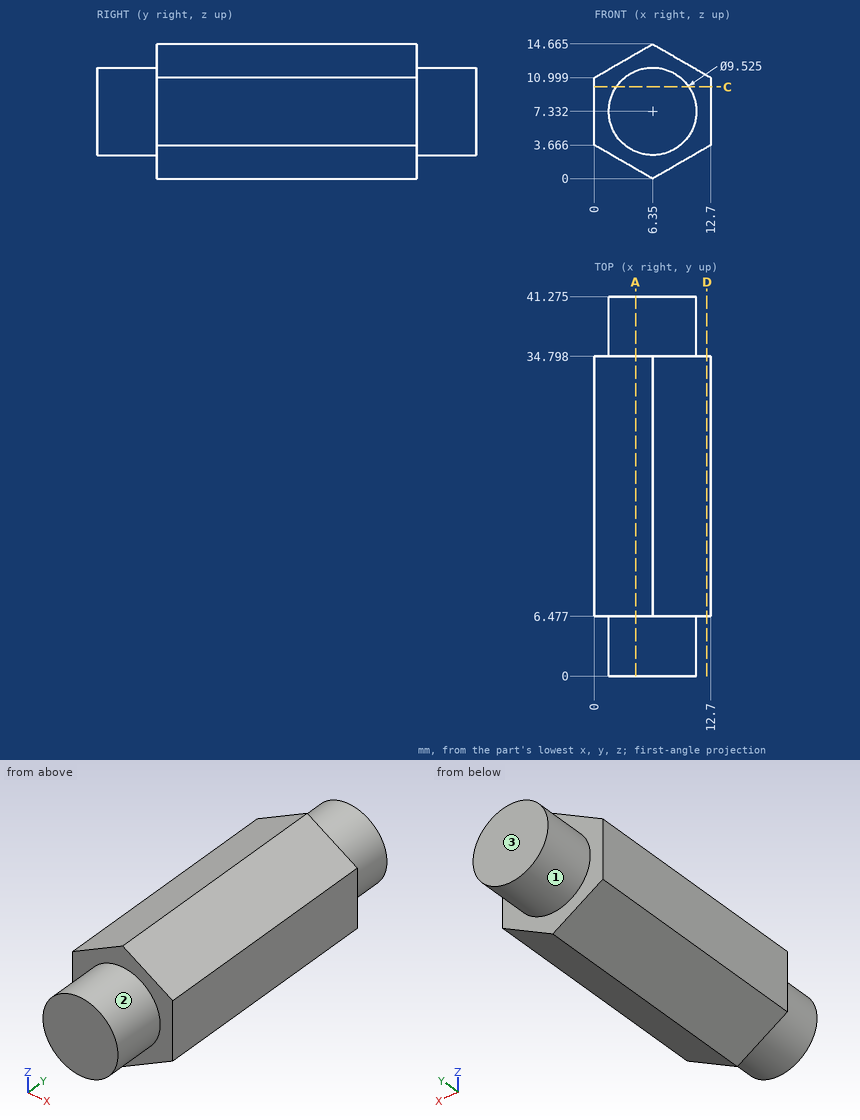
Design review of the part shown in the three views and the two pictorial views. Dimensions are in mm from the part's minimum x, y and z. A direction names the side the tool comes from. Round coordinates to 2 decimals unless told otherwise and drop trailing zeros. Order: outer loops, then holes, each group sorted by start corner. A loop starts at its lowest first (then second) coordinate and runs counter-clockwise, first axis right, second up.
Q1. Insertion check: P1, Ø5, axis at x = 2, y = 33.5, coming from the +Z side; P2, Ø2, axis at x = 2.5, y = 26.5, coming from the -Z side (1 decimal). Each pin has a flat end and moves straight along its axis. Give the tip position at first contact, or say it passes through.
Findings below:
P1: stops at z = 13.6
P2: stops at z = 1.6
Q2. We need section A-A, the plane x = 4.5. Give the boundary of the cut face in (y, z) (1 decimal).
Findings below:
outline: (0, 2.9) - (6.5, 2.9) - (6.5, 1.1) - (34.8, 1.1) - (34.8, 2.9) - (41.3, 2.9) - (41.3, 11.7) - (34.8, 11.7) - (34.8, 13.6) - (6.5, 13.6) - (6.5, 11.7) - (0, 11.7) - close
Q3. Machinability: for the marked faces 1, 2 and 3, which of the approach directions +Z, -Z, +X, -X, +Y, -Y give a long, thin tool a straight path to every point of the face, cutting with its end or side? Answer none if there is none.
Findings below:
face 1: +Y
face 2: -Y
face 3: +Z, -Z, +X, -X, +Y
Q4. We need section D-D, the plane x = 12.25. Give the boundary of the cut face in (y, z).
Findings below:
outline: (6.48, 3.41) - (34.8, 3.41) - (34.8, 11.26) - (6.48, 11.26) - close
Q5. We need section C-C, the plane z = 10. Give the boundary of the cut face in (x, y) (1 decimal).
Findings below:
outline: (0, 6.5) - (2.4, 6.5) - (2.4, 0) - (10.3, 0) - (10.3, 6.5) - (12.7, 6.5) - (12.7, 34.8) - (10.3, 34.8) - (10.3, 41.3) - (2.4, 41.3) - (2.4, 34.8) - (0, 34.8) - close
Q6. Wall thickness on line 1 (Y direction, x = 12, z = 8.75); line 2 (Z direction, x = 4.75, y = 15) (1 decimal); line 3 (Z direction, x = 11, y = 33.5) (1 decimal): over which ranges is each line inside the solid? List them lowest first.
Findings below:
line 1: y = 6.48 to 34.8
line 2: z = 0.9 to 13.7
line 3: z = 2.7 to 12
